Autodesk Inventor part; units mm, degrees
ref_plane "YZ Plane" through (0, 0, 0) normal (1, 0, 0) x (0, 1, 0)
ref_plane "XZ Plane" through (0, 0, 0) normal (0, 1, 0) x (-1, 0, 0)
ref_plane "XY Plane" through (0, 0, 0) normal (0, 0, 1) x (1, 0, 0)
sketch "Sketch1" plane through (0, 0, 0) normal (0, 0, 1) x (1, 0, 0)
  line L0 (-180, 0) -> (0, 0)
  line L1 (-225, -45) -> (0, -45)
  line L2 (-180, 0) -> (-225, -45)
  line L3 (0, 0) -> (0, -45)
  dimension "d2" = 45
  dimension "d9" = 225
  dimension "d10" = 180
extrude "Extrusion1" add sketch "Sketch1" along normal blind 10
sketch "Sketch4" plane through (0, 0, 0) normal (0, 0, -1) x (-1, 0, 0)
  circle A0 centre (22.5, -22.5) radius 7.5
  circle A1 centre (157.5, -22.5) radius 7.5
  point P0 (0, -45)
  point P1 (180, 0)
  dimension "d26" = 15
  dimension "d30" = 15
extrude "Extrusion2" add sketch "Sketch4" along normal blind 10
fillet "Fillet5" radius 5 2 edges at (-225, -45, 5) (-180, 0, 5)
chamfer "Chamfer3" distance 2 angle 45 5 edges at (-106.4645, -45, 10) (-217.5483, -41.9134, 10) (-198.9645, -18.9645, 10) (-179.8423, -0.3806, 10) (-88.9645, 0, 10)
mirror "Mirror1" about plane through (0, 0, 0) normal (1, 0, 0)
sketch "Sketch6" plane through (0, 0, 10) normal (0, 0, 1) x (1, 0, 0)
  line L0 (0, 20) -> (-220, 20)
  line L1 (-220, 20) -> (-220, -60)
  line L2 (-220, -60) -> (0, -60)
  line L3 (0, -60) -> (0, 20)
  point P0 (0, 0)
  dimension "d47" = 220
  dimension "d48" = 80
extrude "Extrusion6" cut sketch "Sketch6" against normal blind 20
properties part number "Border"
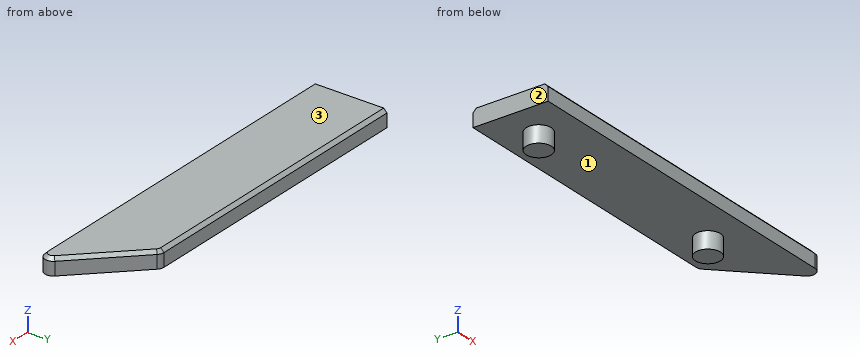
Model file for the job. Use its own axes, mm. Face numbers are marked on the shaded views. Give positions to 0.01 mm unless a question says otherwise; leave off trailing zeros. Loops run counter-clockwise (first coordinate to the right, second up) from the corner with the lowest first, then second, coordinate; pieces in that order, holes last.
1) Saw through at B-B (z = 4.5). Write the cut outline in (x, y).
2) Saw through at D-D (x = 137). Write the cut outline in (y, z).
3) Flat gauge pins, fed straight in: pin 1 Ø6 at (x, y) = (76.5, -18) entering from -Z; pin 2 Ø8 at (x, y) = (150.5, -18.5) entering from -Z; pin 3 Ø8 at (y, z) = (-27, 0) entering from +X; pin 4 Ø8 at (y, z) = (-16.5, -4.5) entering from -X. Where does each tip first touch, or does it go through?
4) Pull direction X, two halves, no side cores. Call the marked faces 1, 2 and 3: +X half, -X half, draft (parallel to the pull), parting line (faces both ways), or undercut.
5) Wall check: line 1 (Z direction, x = 38, y = -3.5); line 2 (X direction, y = -16, z = -2); line 3 (X direction, y = -1.5, z = 1.5). Give the ranges that are in metal, low to high.
6) Saw through at C-C (y = -20). Write the cut outline in (x, z).
7) Saw through at A-A (x = 22.5). Write the cut outline in (y, z).
Answer block:
1. outline: (0, -45) - (212.93, -45) arc R5 ccw to (216.46, -36.46) - (181.46, -1.46) arc R5 ccw to (177.93, 0) - (0, 0) - close
2. outline: (-45, 0) - (0, 0) - (0, 8) - (-2, 10) - (-43, 10) - (-45, 8) - close
3. pin 1: stops at z = 0
3. pin 2: stops at z = -10
3. pin 3: stops at x = 211
3. pin 4: stops at x = 15.27
4. face 1: undercut
4. face 2: -X half
4. face 3: draft
5. line 1: z = 0 to 10
5. line 2: x = 18.76 to 26.24, 153.76 to 161.24
5. line 3: x = 0 to 181.5
6. outline: (0, 0) - (15.43, 0) - (15.43, -10) - (29.57, -10) - (29.57, 0) - (150.43, 0) - (150.43, -10) - (164.57, -10) - (164.57, 0) - (200, 0) - (200, 8) - (197.17, 10) - (0, 10) - close
7. outline: (-45, 0) - (-30, 0) - (-30, -10) - (-15, -10) - (-15, 0) - (0, 0) - (0, 8) - (-2, 10) - (-43, 10) - (-45, 8) - close
